from build123d import *

# Parameters (mm, degrees)
F1_DEPTH = 11
F2_DEPTH = 5
F0_R     = 10.5
F3_DEPTH = 11
F0_R_2   = 15
F0_R_3   = 22
F4_DEPTH = 20
F6_DEPTH = 40.001
F0_R_4   = 4
F7_DEPTH = 16


with BuildPart() as f1:
    # F0 (on Top) → F1 (new body, symmetric)
    with BuildSketch(Plane.XY):
        with BuildLine():
            ThreePointArc((30, 0), (27.672658, -15.077059), (20.907291, -28.75054))
            Line((20.907291, -28.75054), (100.377335, 84.322267))
            ThreePointArc((100.377335, 84.322267), (91.78917, 76.692756), (80.695661, 73.709459))
            ThreePointArc((80.695661, 73.709459), (76.907348, 73.880171), (73.188437, 74.621899))
            ThreePointArc((73.188437, 74.621899), (76.550642, 71.486924), (75.932116, 66.931717))
            Line((75.932116, 66.931717), (37.831971, 12.721475))
            ThreePointArc((37.831971, 12.721475), (37.189959, 11.459233), (36.219799, 10.42762))
            ThreePointArc((36.219799, 10.42762), (31.542706, 9.582736), (28.272027, 13.03117))
            ThreePointArc((28.272027, 13.03117), (29.566124, 6.572619), (30, 0))
        make_face()
        with BuildLine():
            ThreePointArc((-105.684211, -17.571067), (-118.841538, -27.847598), (-135.454545, -29.499965))
            Line((-135.454545, -29.499965), (-29.090909, -49.166608))
            ThreePointArc((-29.090909, -49.166608), (-49.187749, -40.596494), (-63.711715, -24.275212))
            ThreePointArc((-63.711715, -24.275212), (-64.023238, -29.621509), (-68.991978, -31.619394))
            Line((-68.991978, -31.619394), (-102.54067, -25.416239))
            ThreePointArc((-102.54067, -25.416239), (-106.272846, -22.359322), (-105.684211, -17.571067))
        make_face()
        with BuildLine():
            Line((-42.434373, 46.699401), (-135.454545, 29.499965))
            ThreePointArc((-135.454545, 29.499965), (-118.841538, 27.847598), (-105.684211, 17.571067))
            ThreePointArc((-105.684211, 17.571067), (-106.272846, 22.359322), (-102.54067, 25.416239))
            Line((-102.54067, 25.416239), (-68.991978, 31.619394))
            ThreePointArc((-68.991978, 31.619394), (-64.023238, 29.621509), (-63.711715, 24.275212))
            ThreePointArc((-63.711715, 24.275212), (-60.527668, 29.283239), (-56.772692, 33.878741))
            ThreePointArc((-56.772692, 33.878741), (-33.707162, 48.084443), (-6.618193, 48.176003))
            ThreePointArc((-6.618193, 48.176003), (-10.007535, 51.365559), (-9.30078, 55.965711))
            ThreePointArc((-9.30078, 55.965711), (-8.098503, 57.123507), (-6.582138, 57.821073))
            Line((-6.582138, 57.821073), (48.105951, 95.143458))
            ThreePointArc((48.105951, 95.143458), (52.669238, 95.699243), (55.757649, 92.294218))
            ThreePointArc((55.757649, 92.294218), (55.098399, 95.747126), (54.929981, 99.258368))
            ThreePointArc((54.929981, 99.258368), (57.950504, 110.621425), (65.831236, 119.347059))
            Line((65.831236, 119.347059), (-37.851813, 48.587617))
            ThreePointArc((-37.851813, 48.587617), (-40.044545, 47.404341), (-42.434373, 46.699401))
        make_face()
    extrude(amount=F1_DEPTH, both=True)



with BuildPart() as f2:
    # F0 (on Top) → F2 (new body, symmetric)
    with BuildSketch(Plane.XY):
        with BuildLine():
            ThreePointArc((-100, 0), (-101.456405, -9.233805), (-105.684211, -17.571067))
            ThreePointArc((-105.684211, -17.571067), (-106.272846, -22.359322), (-102.54067, -25.416239))
            Line((-102.54067, -25.416239), (-68.991978, -31.619394))
            ThreePointArc((-68.991978, -31.619394), (-64.023238, -29.621509), (-63.711715, -24.275212))
            ThreePointArc((-63.711715, -24.275212), (-70, 0), (-63.711715, 24.275212))
            ThreePointArc((-63.711715, 24.275212), (-64.023238, 29.621509), (-68.991978, 31.619394))
            Line((-68.991978, 31.619394), (-102.54067, 25.416239))
            ThreePointArc((-102.54067, 25.416239), (-106.272846, 22.359322), (-105.684211, 17.571067))
            ThreePointArc((-105.684211, 17.571067), (-101.456405, 9.233805), (-100, 0))
        make_face()
        with BuildLine():
            ThreePointArc((-6.618193, 48.176003), (15.483639, 35.226572), (28.272027, 13.03117))
            ThreePointArc((28.272027, 13.03117), (31.542706, 9.582736), (36.219799, 10.42762))
            Line((36.219799, 10.42762), (37.831971, 12.721475))
            Line((37.831971, 12.721475), (75.932116, 66.931717))
            ThreePointArc((75.932116, 66.931717), (76.550642, 71.486924), (73.188437, 74.621899))
            ThreePointArc((73.188437, 74.621899), (62.124808, 81.141917), (55.757649, 92.294218))
            ThreePointArc((55.757649, 92.294218), (52.669238, 95.699243), (48.105951, 95.143458))
            Line((48.105951, 95.143458), (-6.582138, 57.821073))
            Line((-6.582138, 57.821073), (-9.30078, 55.965711))
            ThreePointArc((-9.30078, 55.965711), (-10.007535, 51.365559), (-6.618193, 48.176003))
        make_face()
    extrude(amount=F2_DEPTH, both=True)


with BuildPart() as f1_1:
    add(f1.part)

    add(f2.part)  # F3 merges F2
    # F0 (on Top) → F3 (join, symmetric)
    with BuildSketch(Plane.XY):
        with BuildLine():
            ThreePointArc((80.695661, 73.709459), (91.78917, 76.692756), (100.377335, 84.322267))
            ThreePointArc((100.377335, 84.322267), (97.722572, 116.253157), (65.831236, 119.347059))
            ThreePointArc((65.831236, 119.347059), (57.950504, 110.621425), (54.929981, 99.258368))
            ThreePointArc((54.929981, 99.258368), (55.098399, 95.747126), (55.757649, 92.294218))
            ThreePointArc((55.757649, 92.294218), (62.124808, 81.141917), (73.188437, 74.621899))
            ThreePointArc((73.188437, 74.621899), (76.907348, 73.880171), (80.695661, 73.709459))
        make_face()
        with Locations((79.92369, 98.697537)):
            Circle(F0_R, mode=Mode.SUBTRACT)
    extrude(amount=F3_DEPTH, both=True)

    # F0 (on Top) → F4 (join, symmetric)
    with BuildSketch(Plane.XY):
        with BuildLine():
            ThreePointArc((-135.454545, 29.499965), (-160, 0), (-135.454545, -29.499965))
            ThreePointArc((-135.454545, -29.499965), (-118.841538, -27.847598), (-105.684211, -17.571067))
            ThreePointArc((-105.684211, -17.571067), (-101.456405, -9.233805), (-100, 0))
            ThreePointArc((-100, 0), (-101.456405, 9.233805), (-105.684211, 17.571067))
            ThreePointArc((-105.684211, 17.571067), (-118.841538, 27.847598), (-135.454545, 29.499965))
        make_face()
        with Locations((-130, 0)):
            Circle(F0_R_2, mode=Mode.SUBTRACT)
        with BuildLine():
            ThreePointArc((-63.711715, -24.275212), (-49.187749, -40.596494), (-29.090909, -49.166608))
            ThreePointArc((-29.090909, -49.166608), (-1.098294, -46.289583), (20.907291, -28.75054))
            ThreePointArc((20.907291, -28.75054), (27.672658, -15.077059), (30, 0))
            ThreePointArc((30, 0), (29.566124, 6.572619), (28.272027, 13.03117))
            ThreePointArc((28.272027, 13.03117), (15.483639, 35.226572), (-6.618193, 48.176003))
            ThreePointArc((-6.618193, 48.176003), (-33.707162, 48.084443), (-56.772692, 33.878741))
            ThreePointArc((-56.772692, 33.878741), (-60.527668, 29.283239), (-63.711715, 24.275212))
            ThreePointArc((-63.711715, 24.275212), (-70, 0), (-63.711715, -24.275212))
        make_face()
        Circle(F0_R_3, mode=Mode.SUBTRACT)
    extrude(amount=F4_DEPTH, both=True)

    # F5 (on face) → F6 (cut, through all)
    with BuildSketch(Plane.XY.offset(20)):
        with BuildLine():
            ThreePointArc((-1.5625, 24.951124), (2.980616, 28.748457), (0.714286, 34.218684))
            ThreePointArc((0.714286, 34.218684), (-34.403073, 37.316906), (-58.332594, 11.428571))
            ThreePointArc((-58.332594, 11.428571), (-57.549938, 7.011928), (-53.54102, 5))
            Line((-53.54102, 5), (-28.284271, 5))
            ThreePointArc((-28.284271, 5), (-25.39752, 5.917517), (-23.570226, 8.333333))
            ThreePointArc((-23.570226, 8.333333), (-15.0649, 19.95116), (-1.5625, 24.951124))
        make_face()
        with BuildLine():
            ThreePointArc((-23.570226, -8.333333), (-25.39752, -5.917517), (-28.284271, -5))
            Line((-28.284271, -5), (-53.54102, -5))
            ThreePointArc((-53.54102, -5), (-57.549938, -7.011928), (-58.332594, -11.428571))
            ThreePointArc((-58.332594, -11.428571), (-34.403073, -37.316906), (0.714286, -34.218684))
            ThreePointArc((0.714286, -34.218684), (2.980616, -28.748457), (-1.5625, -24.951124))
            ThreePointArc((-1.5625, -24.951124), (-15.0649, -19.95116), (-23.570226, -8.333333))
        make_face()
    extrude(amount=-F6_DEPTH, mode=Mode.SUBTRACT)

    # F0 (on Top) → F7 (join, symmetric)
    with BuildSketch(Plane.XY):
        Circle(F0_R_3)
        with Locations((3.337814, -14.623919)):
            Circle(F0_R_4, mode=Mode.SUBTRACT)
        with Locations((-9.352347, -11.727472)):
            Circle(F0_R_4, mode=Mode.SUBTRACT)
        with Locations((-15, 0)):
            Circle(F0_R_4, mode=Mode.SUBTRACT)
        with Locations((-9.352347, 11.727472)):
            Circle(F0_R_4, mode=Mode.SUBTRACT)
        with Locations((3.337814, 14.623919)):
            Circle(F0_R_4, mode=Mode.SUBTRACT)
        with Locations((13.514533, -6.508256)):
            Circle(F0_R_4, mode=Mode.SUBTRACT)
        with Locations((13.514533, 6.508256)):
            Circle(F0_R_4, mode=Mode.SUBTRACT)
    extrude(amount=F7_DEPTH, both=True)


solid = f1_1.part
Input: part model. Units: mm. Frame: model coordinates. A direction names the side the tool comes from. Give positions to 0.01 mm unless a question says otherwise; leave off trailing zeros. Order: outer loops, then holes, each group sorted by start corner. A loop starts at its lowest first (then second) coordinate and runs counter-clockwise, first axis right, second up. Notation, with made-up numbers: (44, 64) - (74, 64) arc R24 ccw to (74, 90) - close; hole circle Ø5 at (-29, 52). An arc over 180 degrees is marked (long way). Write each question's results on one line, items separated by ' | '.
Item 1: Section A-A (x = -130). Return loops of the section in (y, z).
A:
outline: (-30.51, -11) - (-30, -11) - (-30, -20) - (-15, -20) - (-15, 20) - (-30, 20) - (-30, 11) - (-30.51, 11) - close; (15, -20) - (30, -20) - (30, -11) - (30.51, -11) - (30.51, 11) - (30, 11) - (30, 20) - (15, 20) - close
Item 2: Section C-C (x = -80.5). Return loops of the section in (y, z), and give its area (3 significant figures).
A:
outline: (-39.66, -11) - (-29.49, -11) - (-29.49, -5) - (29.49, -5) - (29.49, -11) - (39.66, -11) - (39.66, 11) - (29.49, 11) - (29.49, 5) - (-29.49, 5) - (-29.49, 11) - (-39.66, 11) - close | area: 1,040 mm^2
Item 3: Access query for faces 1 (the flat face through (-83, -34, 11)), 2 (the cylindrical face through (29.58, 6.48, -15.44)), 3 (the cylindrical face through (-106.25, -22.42, 7.96)), 4 (the cylindrical face through (3, -28.83, 0.28)). Directions: +Z, -Z, +X, -X, +Y, -Y. A direction counts if a zero-diameter tool reaches every point of the face in a straight line with its end or side. Return the directions, or none.
A:
face 1: +Z, -Y | face 2: -Z, +X, +Y | face 3: +Z | face 4: +Z, -Z
Item 4: Draft query along Y for faces 5 (the flat face through (-124, 14, 20)), 6 (the flat face through (33, 53, -5)), 7 (the flat face through (14.715, 84.463, 0.154)), 8 (the cylindrical face through (98.061, 115.903, 0.154)). Return one class per face: released by +Y, released by -Y, zero draft, split by the parting line, or undercut.
A:
face 5: zero draft | face 6: undercut | face 7: released by +Y | face 8: split by the parting line
Item 5: Material intervals for line 1 along X through (y, z) = (-5.5, -4); line 2 along Y through (x, z) = (-15, 5); line 3 along X through (y, z) = (-20, 7.5), sorted ascending.
A:
line 1: x = -159.49 to -143.96, -116.04 to -55.72, -26.1 to 9.64, 17.39 to 37.25 | line 2: y = -49.75 to -39.69, -20 to -4, 4 to 20, 39.69 to 64.18 | line 3: x = -152.36 to -106.61, -65.83 to -54.64, -15 to 27.06
Item 6: Contact query for flat-ended pins moving along their axis: pin 1 Ø2 at (x, z) = (-112, 8.5) entering from +Y; pin 2 Ø6 at (x, z) = (-91, -11.5) entering from -Y; pin 3 Ø6 at (y, z) = (77.5, 4) entering from -X. Output: stop coordinate, or through.
A:
pin 1: stops at y = 34.02 | pin 2: stops at y = -38.27 | pin 3: stops at x = 0.12
Item 7: Section B-B (x = 83.5). Return loops of the section in (y, z).
A:
outline: (60.31, -11) - (88.83, -11) - (88.83, 11) - (60.31, 11) - close; (108.57, -11) - (123.44, -11) - (123.44, 11) - (108.57, 11) - close
